Can you work these out from the model? Positions are in its coordinate system, mm. Give positions to 0.01 mm unless a question says otherwise; leave off trailing zeros. Write each loop counter-clockwise with the first axis right and the second up, starting at its lowest first coordinate (ties: lowest second). Pieces come first, ordered by that corner, then holes.
Autodesk Inventor part; units mm, degrees
ref_plane "YZ Plane" through (0, 0, 0) normal (1, 0, 0) x (0, 1, 0)
ref_plane "XZ Plane" through (0, 0, 0) normal (0, 1, 0) x (-1, 0, 0)
ref_plane "XY Plane" through (0, 0, 0) normal (0, 0, 1) x (1, 0, 0)
sketch "Sketch1" plane through (0, 0, 0) normal (0, 0, 1) x (1, 0, 0)
  line L0 (-750, 0) -> (750, 0) construction
  line L1 (750, 0) -> (750, -2700) construction
  line L2 (750, -2700) -> (-750, -2700) construction
  line L3 (-750, -2700) -> (-750, 0) construction
  line L4 (800, 50) -> (-800, 50) construction
  line L5 (-800, 50) -> (-800, -2750) construction
  line L6 (-800, -2750) -> (800, -2750) construction
  line L7 (800, -2750) -> (800, 50) construction
  line L8 (-850, 100) -> (850, 100) construction
  line L9 (850, 100) -> (850, -2800) construction
  line L10 (850, -2800) -> (-850, -2800) construction
  line L11 (-850, -2800) -> (-850, 100) construction
  arc A0 (750, 0) -> (745.2706, 0.6314) centre (0, -5600) ccw construction
  line L12 (-750, -2100) -> (750, -2100) construction
  line L13 (114.1118, -2698.3696) -> (750, -2100) construction
  arc A1 (750, -2100) -> (771.0671, -250.888) centre (-10250, -1050) ccw construction
  line L14 (750, 0) -> (749.6018, -2.9735) construction
  arc A2 (750, -3.0268) -> (0, 47) centre (-0.2, -5603) ccw
  line L15 (750, 0) -> (747.0136, -0.2851) construction
  arc A3 (768.075, -251.105) -> (747.4657, -5.0326) centre (-10252.9897, -1050.251) ccw construction
  arc A4 (750.4522, -4.7486) -> (745.2706, 0.6314) centre (744.4791, -5.3162) ccw construction
  arc A5 (747.4657, -5.0326) -> (744.8748, -2.3426) centre (744.4792, -5.3164) ccw construction
  line L16 (750, -2100) -> (752.9864, -2100.2851) construction
  arc A6 (752.9864, -2100.2851) -> (772.2226, -225.7318) centre (-10246.9893, -1050.0309) ccw construction
  line L17 (750, -2100) -> (752.0559, -2102.1848) construction
  line L18 (752.0559, -2102.1848) -> (752.0559, -2102.1848) construction
  arc A7 (749.1768, -2100.7746) -> (750.1074, -2098.8746) centre (747.1209, -2098.5898) ccw construction
  line L19 (0, -2697) -> (110, -2697) construction
  line L20 (112.0559, -2696.1848) -> (676.8655, -2164.7001) construction
  arc A8 (110, -2700) -> (114.1118, -2698.3696) centre (110, -2694) ccw construction
  arc A9 (110, -2697) -> (112.0559, -2696.1848) centre (110, -2694) ccw construction
  line L21 (676.8655, -2164.7001) -> (678.9214, -2166.8849) construction
  line L22 (752.0559, -2102.1848) -> (662.7706, -2186.2021) construction
  line L23 (662.7706, -2186.2021) -> (660.7147, -2184.0173) construction
  arc A10 (747.4657, -5.0326) -> (747.0136, -0.2851) centre (-10252.9897, -1050.251) ccw construction
  arc A11 (745.2706, 0.6314) -> (0, 50) centre (0, -5600) ccw construction
  arc A12 (750.4522, -4.7486) -> (750, 0) centre (-10250, -1050) ccw construction
  line L24 (771.0671, -250.888) -> (768.075, -251.105) construction
  line L25 (769.231, -225.9556) -> (772.2226, -225.7318) construction
  arc A13 (771.0671, -250.888) -> (750.4522, -4.7486) centre (-10250, -1050) ccw construction
  line L26 (0, 100) -> (0, 50) construction
  line L27 (0, -2700) -> (0, -2697) construction
  line L28 (0, 47) -> (0, 0) construction
  line L29 (0, 50) -> (0, 47) construction
  arc A14 (752.0559, -2102.1848) -> (752.9864, -2100.2851) centre (749.9998, -2099.9999) ccw construction
  line L30 (0, 47) -> (0, -50)
  line L31 (0, -50) -> (751.6456, -50)
  circle A15 centre (450, -15) radius 25
  arc A16 (0, -40) -> (0, 10) centre (0, -15) ccw
  line L32 (747.7149, -7.6588) -> (742.2399, -1.9927)
  line L33 (751.4456, -50) -> (747.5149, -7.4518)
  point P0 (0, -2750)
  point P1 (0, 48.5)
  point P2 (747.2399, -2.6588)
  dimension "d85" = 40
  dimension "d54" = 1500
  dimension "d55" = 2700
  dimension "d58" = 2100
  dimension "d68" = 6
  dimension "d70" = 3
  dimension "d75" = 3
  dimension "d83" = 6
  dimension "d86" = 3
  dimension "d112" = 251.771
  dimension "d113" = 50
  dimension "d114" = 50
  dimension "d115" = 3
  dimension "d117" = 110
  dimension "d118" = 25
  dimension "d119" = 122.6
  dimension "d120" = 25
  dimension "d121" = 50
  dimension "d122" = 50
  dimension "d123" = 450
  dimension "d124" = 35
  dimension "d126" = 98.5
  dimension "d127" = 5
  dimension "d128" = 5
  dimension "d132" = 0.2
  dimension "d133" = 0.2
extrude "Plate3" add sketch "Sketch1" along normal blind 3 contours L32 L33 L31 L30 A16 A2
mirror "Mirror3" about plane through (0, 0, 0) normal (1, 0, 0)
chamfer "Corner Chamfer2" distance 2 angle 45 1 edges at (751.4456, -50, 1.5)
equation "\"BendRadius\" = Thickness"
equation "\"BendReliefWidth\" = Thickness"
equation "\"BendReliefDepth\" = 0.5 * Thickness"
equation "\"CornerReliefSize\" = 4 * Thickness"
equation "\"MinimumRemnant\" = 2 * Thickness"
equation "\"TransitionRadius\" = BendRadius"
equation "\"JacobiRadiusSize\" = BendRadius"
equation "\"GapSize\" = Thickness"
properties part number "MSC 208 sheet back mould" material "Stainless Steel AISI 304"
1) Suppose I cut it at A-A on x = -450. Write out the boundary of the cut face in (y, z).
Values follow:
outline: (-50, 0) - (-40, 0) - (-40, 3) - (-50, 3) - close; (10, 0) - (29.04, 0) - (29.04, 3) - (10, 3) - close
2) Suppose I cut it at D-D on x = -238. Write out the boundary of the cut face in (y, z).
Values follow:
outline: (-50, 0) - (41.98, 0) - (41.98, 3) - (-50, 3) - close
3) Please list where these lines run through material, in increasing order: L1, parallel to X at y = -16, z = 1.6; L2, parallel to Y at x = 0, z = 0.85; L3, parallel to X at y = -25, z = 2.7.
Values follow:
L1: x = -748.3 to -474.98, -425.02 to -24.98, 24.98 to 425.02, 474.98 to 748.3
L2: y = -50 to -40, 10 to 47
L3: x = -749.14 to -472.91, -427.09 to -22.91, 22.91 to 427.09, 472.91 to 749.14
4) Suppose I cut it at B-B on z = 2.5. Write out the boundary of the cut face in (x, y).
Values follow:
outline: (-751.45, -50) - (749.45, -50) - (751.26, -48.01) - (747.51, -7.45) - (742.24, -1.99) arc R5650 ccw to (0, 47) arc R5650 ccw to (-742.24, -1.99) - (-747.51, -7.45) - close; hole circle Ø50 at (-450, -15); hole circle Ø50 at (0, -15); hole circle Ø50 at (450, -15)
5) If we mould it in two halves opening along X, with no side actions, what happens to faces 1 (the face through (-11, 10, 0)), 2 (the face through (15, 5, 1))? For each: +X half, -X half, draft (parallel to the pull), parting line (faces both ways), or undercut.
Values follow:
face 1: draft
face 2: undercut
6) Suppose I cut it at C-C on x = 494. Write out the boundary of the cut face in (y, z).
Values follow:
outline: (-50, 0) - (25.34, 0) - (25.34, 3) - (-50, 3) - close
